Geometry: final body of the model. Coordinates: model frame, mm. A direction names the side the tool comes from. Round coordinates to 2 decimals unless told otherwise and drop trailing zeros. Write each loop counter-clockwise with the first axis right and the second up, starting at its lowest first coordinate (ties: lowest second). Pieces come first, ordered by that corner, then holes. Notation, with made-up numbers: (44.25, 36.5) -> (63.25, 36.5) arc R18 ccw to (63.25, 59.5) -> close; hole circle Ø5 at (-4.5, -13). An arc over 180 degrees is marked (long way). Use one line per item in the form item = value. Start each with the question number.
1. Cut plane A-A, the plane y = 42. Return the cut outline in (x, z), plus the area to 3 significant figures.
2. Line query: L1, parallel to Y at x = 9, z = 2.5; L2, parallel to Y at x = 20, z = 4; L3, parallel to X at y = 45.5, z = -3.5. Output: solid intervals per line, ascending.
3. Draft query along Y for faces 1 (the face through (12, 35, 0.5)), 2 (the face through (21.59, 49.19, -2.94)), 3 (the face through (25, 39, -0.2)), 4 (the face through (8.34, 46.59, -1.57)). Return one class per face: pulls with the +Y half, pulls with the -Y half, needs draft (parallel to the pull), parting line crosses it, or undercut.
4. Cut plane D-D, the plane z = 1. Return the cut outline in (x, y).
5. Cut plane B-B, the plane x = 15. State how many separate pieces and enclosed holes the cut face has, plus the area to 3 significant figures.
6. Pin query (flat end, axial travel): pin 1 Ø6 at (y, z) = (51.5, -0.5) entering from +X; pin 2 Ø1.7 at (x, z) = (15, -2.81) entering from +Y; pin 3 Ø8 at (x, y) = (16.5, 37.5) entering from +Z. Return the tip coordinate at first contact, or that it passes through.
7. Reachability of faces 5 (the face through (15.303, 33.933, -1.447)), 6 (the face through (14, 52, 3)), 7 (the face through (1.33, 45.03, 2.69)) from +Z, -Z, +X, -X, +Y, -Y: full face, straight path, thin tool, end or side. Return the list, or none.
8. Cut plane C-C, the plane z = -2. Return the cut outline in (x, y).
Autodesk Inventor part; units mm, degrees
ref_plane "YZ Plane" through (0, 0, 0) normal (1, 0, 0) x (0, 1, 0)
ref_plane "XZ Plane" through (0, 0, 0) normal (0, 1, 0) x (-1, 0, 0)
ref_plane "XY Plane" through (0, 0, 0) normal (0, 0, 1) x (1, 0, 0)
ref_plane "Arbeitsebene1" through (15, 0, 0) normal (-1, 0, 0) x (0, 1, 0)
sketch "Skizze1" plane through (15, 0, 0) normal (-1, 0, 0) x (0, 1, 0)
  line L0 (32.6031, 0.5) -> (30.7237, 0.5)
  line L1 (30.7237, 4.25) -> (32.6031, 4.25)
  line L2 (30.7237, 0.5) -> (30.7237, 4.25)
  line L3 (32.6031, 0.5) -> (30.7237, 0.5)
  line L4 (30.7237, 4.7) -> (32.6031, 4.7)
  line L5 (30.7237, 0.5) -> (30.7237, 4.25)
  line L6 (30, 0.5) -> (32, 0.5)
  line L7 (30, 0.55) -> (30, 0.5)
  line L8 (32, 0.5) -> (32, 0.55)
  line L9 (32, 0.5) -> (32, 16.1)
  line L10 (52, 0.5) -> (52, 16.1)
  line L11 (42, 19.32) -> (42, -3.22)
  line L12 (32.6031, 0.5) -> (28, 0.5)
  line L13 (28, 0.5) -> (28, -5.5)
  line L14 (28, -5.5) -> (35.6031, -5.5)
  line L15 (35.6031, -5.5) -> (35.6031, 5.25)
  line L16 (35.6031, 5.25) -> (34.1031, 5.25)
  line L17 (32.6031, 0.5) -> (32.6031, 0.2)
  line L18 (32.6031, 0.2) -> (28, 0.2)
  line L19 (32, 0.55) -> (30, 0.55)
  line L20 (32.1031, 0.5) -> (32.0412, 0.2)
  line L21 (28, -5.5) -> (32, -5.5)
  line L22 (32, -5.5) -> (32, -13.5)
  line L23 (32, -13.5) -> (28, -13.5)
  line L24 (28, -13.5) -> (28, -5.5)
  line L25 (34.1031, 5.25) -> (32.307, 3.9176)
  line L26 (32.307, 3.9176) -> (32.1031, 0.5)
  point P0 (0, 0)
  dimension "d1" = 6
  dimension "d3" = 1
  dimension "d11" = 0.5
  dimension "d13" = 14
  dimension "d14" = 8
  dimension "d15" = 10
  dimension "d37" = 0.3
  dimension "d38" = 6.3969
revolve "Umdrehung1" add sketch "Skizze1" angle 360 about axis through (15, 42, -19.32) along (0, 0, 1) contours L17 L18 L20 L0 | L0 L26 L25 L16 L15 L14 L13 L18 L17
sketch "Skizze2" plane through (0, 0, 0) normal (0, 1, 0) x (-1, 0, 0)
  spline S0 degree 3 poles (-15, -4.25) (-12.1304, -4.4784) (-9.2732, -4.7067) (-7.1109, -4.9351) (-6.8554, -4.962) (-6.6095, -4.989) (-6.3738, -5.016) knots 0 0 0 0 0.7174 0.7174 0.7174 0.802142 0.802142 0.802142 0.802142
  spline S1 degree 3 poles (-14.5016, -1.0897) (-11.6314, -1.3183) (-8.8183, -1.5469) (-6.7355, -1.7755) (-6.2054, -1.8336) (-5.7215, -1.8918) (-5.2918, -1.95) knots 0.041547 0.041547 0.041547 0.041547 0.759706 0.759706 0.759706 0.942478 0.942478 0.942478 0.942478
  circle A0 centre (-15, -2.8138) radius 1.4
  line L0 (-15, 1.0048) -> (-15, -6.0288)
  point P0 (0, 0)
  dimension "d5" = 2.8
extrude "Extrusion1" cut sketch "Skizze2" along normal up to surface
pattern_circular "Runde Anordnung1" count 3 over 360 about axis through (15, 42, 2.65) along (0, 0, -1) of "Extrusion1"
chamfer "Fase1" distance 1 angle 45 1 edges at (15, 48.3969, 5.5)
sketch "Skizze6" plane through (15, 42, 5.5) normal (0, 0, 1) x (1, 0, 0)
  circle A0 centre (0, 0) radius 14
  circle A1 centre (0, 0) radius 7.3969
  circle A2 centre (0, 0) radius 10.05
  point P0 (-15, -42)
  dimension "d31" = 20.1
extrude "Extrusion4" cut sketch "Skizze6" against normal blind 5 contours A1 | A2
chamfer "Fase3" distance 1 angle 45 3 edges at (15, 48.3969, 0.5) (4.95, 42, 5.5) (4.95, 42, 0.5)
properties part number "30_Linear_Stage_NEMA11_baseholder_bayonetmount_objective_v0"
Outcome:
q1.outline = (1, -0.2) -> (5.04, -0.2) -> (5.1, -0.5) -> (5.31, -3.92) -> (7.1, -5.25) -> (8.6, -5.25) -> (8.6, -0.5) -> (7.6, 0.5) -> (5.95, 0.5) -> (4.95, 1.5) -> (4.95, 4.5) -> (3.95, 5.5) -> (1, 5.5) -> close; (21.4, -5.25) -> (22.9, -5.25) -> (24.69, -3.92) -> (24.9, -0.5) -> (24.96, -0.2) -> (29, -0.2) -> (29, 5.5) -> (26.05, 5.5) -> (25.05, 4.5) -> (25.05, 1.5) -> (24.05, 0.5) -> (22.4, 0.5) -> (21.4, -0.5) -> close
q1.area = 80.9 mm^2
q2.L1 = 29.35 to 33.94, 50.06 to 54.65
q2.L2 = 28.92 to 33.28, 50.72 to 55.08
q2.L3 = 5.93 to 6.5, 23.5 to 24.07
q3.face_1 = undercut
q3.face_2 = parting line crosses it
q3.face_3 = needs draft
q3.face_4 = undercut
q4.outline = circle Ø28 at (15, 42); hole circle Ø19.1 at (15, 42)
q5.separate_pieces = 3
q5.enclosed_holes = 0
q5.area = 71.5 mm^2
q6.pin_1 = 27.39
q6.pin_2 = 51.81
q6.pin_3 = 0.5
q7.face_5 = -Y
q7.face_6 = +Z
q7.face_7 = +Z, -Z
q8.outline = (5.99, 45.88) arc R9.81 ccw to (13.86, 32.26) -> (13.86, 35.71) arc R6.4 cw to (8.98, 44.16) -> close; (7.13, 47.86) -> (10.12, 46.13) arc R6.4 cw to (19.88, 46.13) -> (22.87, 47.86) arc R9.81 ccw to start; (16.14, 32.26) arc R9.81 ccw to (24.01, 45.88) -> (21.02, 44.16) arc R6.4 cw to (16.14, 35.71) -> close
